The model under review builds one solid part; all positions refer to its coordinate system, in mm. A direction names the side the tool comes from. Round coordinates to 2 decimals unless told otherwise and drop trailing zeros. Order: outer loops, then holes, each group sorted by start corner. A loop starts at its lowest first (then second) coordinate and runs counter-clockwise, first axis right, second up. Notation, with made-up numbers: (86.5, 70) -> (108.5, 70) arc R22 ccw to (108.5, 84) -> close; hole circle Ø1 at (26.25, 59). An arc over 180 degrees is marked (long way). Use a Markdown table: item, result. Add a question column.
```python
from build123d import *

# Parameters (mm, degrees)
BOSS_EXTRU_1_DEPTH        = 9
ESQUISSE2_W               = 45
ESQUISSE2_H               = 80
ENL_V_MAT_EXTRU_2_DEPTH   = 9
D_GAGEMENT_M31_AT_2_COUNT = 2
D_GAGEMENT_M31_AT_2_PITCH = 24


with BuildPart() as part:
    # Esquisse1 → Boss.-Extru.1 (new body)
    with BuildSketch(Plane(origin=(0, 0, 0), x_dir=(1, 0, 0), z_dir=(0, 1, 0))):
        Polygon((0, 110), (-160, 53.578166916), (-60, -230), (60, -230), (160, 53.578166916), align=None)
    extrude(amount=-BOSS_EXTRU_1_DEPTH)

    # Esquisse2 → Enlèv. mat.-Extru.2 (cut)
    with BuildSketch(Plane(origin=(0, 0, 0), x_dir=(1, 0, 0), z_dir=(0, 1, 0))):
        with Locations((-92.5, 15)):
            Rectangle(ESQUISSE2_W, ESQUISSE2_H)
    enl_v_mat_extru_2 = extrude(amount=-ENL_V_MAT_EXTRU_2_DEPTH, mode=Mode.SUBTRACT)

    # Symétrie1: Enlèv. mat.-Extru.2 across plane
    add(enl_v_mat_extru_2.mirror(Plane(origin=(0, 0, 0), x_dir=(0, 0, 1), z_dir=(1, 0, 0))), mode=Mode.SUBTRACT)

    # Esquisse4 → Dégagement M31 (revolve, cut)
    with BuildSketch(Plane(origin=(-58, 0, 0), x_dir=(0, 0, 1), z_dir=(1, 0, 0))):
        Polygon((0, 0), (0, 11.021463052), (1.7, 10), (1.7, 0), align=None)
    d_gagement_m31 = revolve(axis=Axis((-58, 6.35, 0), (0, -1, 0)), mode=Mode.SUBTRACT)

    # Dégagement M31 at 2: Dégagement M31 ×2
    with Locations(*[(i * D_GAGEMENT_M31_AT_2_PITCH, 0, 0) for i in range(1, D_GAGEMENT_M31_AT_2_COUNT)]):
        add(d_gagement_m31, mode=Mode.SUBTRACT)

    # Symétrie2: Dégagement M31 across plane
    add(d_gagement_m31.mirror(Plane.XY.offset(-15)), mode=Mode.SUBTRACT)

    # Symétrie2 copy 1 sketch → Symétrie2 copy 1 (revolve, cut)
    with BuildSketch(Plane(origin=(-34, 0, -30), x_dir=(0, 0, -1), z_dir=(1, 0, 0))):
        Polygon((0, 0), (0, -11.021463052), (1.7, -10), (1.7, 0), align=None)
    revolve(axis=Axis((-34, 6.35, -30), (0, 1, 0)), mode=Mode.SUBTRACT)

    # Symétrie3: Dégagement M31 across plane
    add(d_gagement_m31.mirror(Plane(origin=(0, 0, 0), x_dir=(0, 0, 1), z_dir=(1, 0, 0))), mode=Mode.SUBTRACT)

    # Symétrie3 copy 1 sketch → Symétrie3 copy 1 (revolve, cut)
    with BuildSketch(Plane(origin=(58, 0, -30), x_dir=(0, 0, -1), z_dir=(-1, 0, 0))):
        Polygon((0, 0), (0, 11.021463052), (1.7, 10), (1.7, 0), align=None)
    revolve(axis=Axis((58, 6.35, -30), (0, -1, 0)), mode=Mode.SUBTRACT)

    # Symétrie3 copy 2 sketch → Symétrie3 copy 2 (revolve, cut)
    with BuildSketch(Plane(origin=(34, 0, -30), x_dir=(0, 0, -1), z_dir=(-1, 0, 0))):
        Polygon((0, 0), (0, 11.021463052), (1.7, 10), (1.7, 0), align=None)
    revolve(axis=Axis((34, 6.35, -30), (0, -1, 0)), mode=Mode.SUBTRACT)

    # Symétrie3 copy 3 sketch → Symétrie3 copy 3 (revolve, cut)
    with BuildSketch(Plane.ZY.offset(-34)):
        Polygon((0, 0), (0, -11.021463052), (1.7, -10), (1.7, 0), align=None)
    revolve(axis=Axis((34, 6.35, 0), (0, 1, 0)), mode=Mode.SUBTRACT)


solid = part.part
```
Q1. Mouldability with a two-part tool opening along X and no side actions: class faces 3 (the flat face through (-93, -4, 25)), 4 (the flat face through (-1, -4, 230)), 5 (the flat face through (81.1, -4.4, -81.4)), 6 (the flat face through (-110.7, -4.44, 86.23)) as pulls with the +X half, pulls with the -X half, needs draft (parallel to the pull), parting line crosses it, or undercut.
Q2. Add section A-A (x = -101.5). Write out the cut boundary in (y, z), then the cut area to 3 significant figures.
Q3. Add section C-C (y = -2.5). State how many separate pieces and enclosed holes the cut face has, then the cut area to 3 significant figures.
Q4. Insertion check: pin 1 (2.5 mm diameter, centred on x = -58, z = 0, fed in from +Y); pin 2 (2.5 mm diameter, centred on y = -6.5, z = -22.5, fed in from +X); pin 3 (5.5 mm diameter, centred on x = -58, z = -30, fed in from +Y); pin 4 (4 mm diameter, centred on y = -2.5, z = 156.5, fed in from -X). Each pin has a flat end and moves straight along its axis. Give the tip position at first contact, or say it passes through.
Q5. Add section B-B (z = -8). Write out the cut boundary in (x, y).
Q6. Machinability: for faces 1 (the flat face through (-78.88, -4.437, -82.184)), 2 (the flat face through (93, -4, -55)), which of the approach directions +Z, -Z, +X, -X, +Y, -Y give a long, thin tool a straight path to every point of the face, cutting with its end or side? Answer none if there is none.
Q7. Add section D-D (x = 99.5). Write out the cut boundary in (y, z).
Q8. Wall thickness on line 1 (Z direction, x = -34, y = -6.25); line 2 (Z direction, x = -58, y = -3); line 3 (X direction, y = -6.25, z = -21.5): over which ranges is each line inside the solid? List them lowest first. Write a range as [from, to].
Report:
| question | item | result |
|---|---|---|
| 1 | face 3 | undercut |
| 1 | face 4 | needs draft |
| 1 | face 5 | pulls with the +X half |
| 1 | face 6 | pulls with the -X half |
| 2 | outline | (-9, -74.21) -> (0, -74.21) -> (0, -55) -> (-9, -55) -> close; (-9, 25) -> (0, 25) -> (0, 112.32) -> (-9, 112.32) -> close |
| 2 | area | 959 mm² |
| 3 | separate pieces | 1 |
| 3 | enclosed holes | 10 |
| 3 | area | 64,100 mm² |
| 4 | pin 1 | passes through |
| 4 | pin 2 | stops at x = 149.48 |
| 4 | pin 3 | stops at y = 0 |
| 4 | pin 4 | stops at x = -86.62 |
| 5 | outline | (-143.93, -9) -> (-115, -9) -> (-115, 0) -> (-143.93, 0) -> close; (-70, -9) -> (70, -9) -> (70, 0) -> (-70, 0) -> close; (115, -9) -> (143.93, -9) -> (143.93, 0) -> (115, 0) -> close |
| 6 | face 1 | -Z, -X, +Y, -Y |
| 6 | face 2 | +Y, -Y |
| 7 | outline | (-9, -74.91) -> (0, -74.91) -> (0, -55) -> (-9, -55) -> close; (-9, 25) -> (0, 25) -> (0, 117.99) -> (-9, 117.99) -> close |
| 8 | line 1 | z = [-98.01, -31.7], [-28.3, -1.7], [1.7, 230] |
| 8 | line 2 | z = [-89.55, -31.7], [-28.3, -1.7], [1.7, 230] |
| 8 | line 3 | x = [-148.69, -115], [-70, 70], [115, 148.69] |
